Input: part model. Units: mm. Frame: model coordinates. A direction names the side the tool comes from. Give positions to 0.01 mm unless a question says otherwise; leave off trailing zeros. Write each loop counter-clockwise with the first axis right and the second up, starting at its lowest first coordinate (ties: lowest second). Pieces come first, ordered by that corner, then holes. Notation, with made-up numbers: (10.25, 41.25) -> (40.25, 41.25) arc R22 ccw to (40.25, 69.25) -> close; hole circle Ø7 at (-31, -18.75). An arc over 180 degrees is marked (long way). Answer as a JSON object with one key per item and string values. Group by question number.
from build123d import *

# Parameters (mm, degrees)
F1_DEPTH = 30
F4_DEPTH = 51.5
F5_DEPTH = 53.5
F6_DEPTH = 45
F7_DEPTH = 3


with BuildPart() as f1:
    # F0 (on Top) → F1 (new body)
    with BuildSketch(Plane.XY):
        with BuildLine():
            Line((92.1, -37.1), (90, -37.1))
            Line((90, -37.1), (70.1, -37.1))
            Line((70.1, -37.1), (55.207107, -37.1))
            Line((55.207107, -37.1), (58.096194, -39.989087))
            ThreePointArc((58.096194, -39.989087), (58.421353, -40.475722), (58.535534, -41.049747))
            Line((58.535534, -41.049747), (58.535534, -41.635534))
            ThreePointArc((58.535534, -41.635534), (58.096194, -42.696194), (57.035534, -43.135534))
            Line((57.035534, -43.135534), (43.964466, -43.135534))
            ThreePointArc((43.964466, -43.135534), (42.903806, -42.696194), (42.464466, -41.635534))
            Line((42.464466, -41.635534), (42.464466, -41.049747))
            ThreePointArc((42.464466, -41.049747), (42.578647, -40.475722), (42.903806, -39.989087))
            Line((42.903806, -39.989087), (45.792893, -37.1))
            Line((45.792893, -37.1), (45, -37.1))
            Line((45, -37.1), (26.284599, -37.1))
            Line((26.284599, -37.1), (29.173687, -39.989087))
            ThreePointArc((29.173687, -39.989087), (29.498846, -40.475722), (29.613026, -41.049747))
            Line((29.613026, -41.049747), (29.613026, -41.635534))
            ThreePointArc((29.613026, -41.635534), (29.173687, -42.696194), (28.113026, -43.135534))
            Line((28.113026, -43.135534), (15.041959, -43.135534))
            ThreePointArc((15.041959, -43.135534), (13.981298, -42.696194), (13.541959, -41.635534))
            Line((13.541959, -41.635534), (13.541959, -41.049747))
            ThreePointArc((13.541959, -41.049747), (13.656139, -40.475722), (13.981298, -39.989087))
            Line((13.981298, -39.989087), (16.870386, -37.1))
            Line((16.870386, -37.1), (12, -37.1))
            Line((12, -37.1), (12, -77.1))
            Line((12, -77.1), (125.1, -77.1))
            Line((125.1, -77.1), (125.1, -37.1))
            Line((125.1, -37.1), (92.1, -37.1))
        make_face()
    extrude(amount=F1_DEPTH)

    # F3 (on offset) → F4 (cut, symmetric)
    with BuildSketch(Plane.YZ.offset(68.5)):
        Polygon((-52.029371, 26.9), (-45.2, 0), (-45.2, 26.9), align=None)
        Polygon((-77.2, 0), (-45.2, 0), (-70.498638, 26.9), (-77.2, 26.9), align=None)
        Polygon((-70.498638, 26.9), (-45.2, 0), (-52.029371, 26.9), align=None)
    extrude(amount=F4_DEPTH, both=True, mode=Mode.SUBTRACT)

    # F3 (on offset) → F5 (join, symmetric)
    with BuildSketch(Plane.YZ.offset(68.5)):
        Polygon((-52.029371, 26.9), (-45.2, 0), (-45.2, 26.9), align=None)
        Polygon((-70.498638, 26.9), (-45.2, 0), (-52.029371, 26.9), align=None)
    extrude(amount=F5_DEPTH, both=True)

    # F3 (on offset) → F6 (cut, symmetric)
    with BuildSketch(Plane.YZ.offset(68.5)):
        Polygon((-70.498638, 26.9), (-45.2, 0), (-52.029371, 26.9), align=None)
    extrude(amount=F6_DEPTH, both=True, mode=Mode.SUBTRACT)

    # F3 (on offset) → F7 (join, symmetric)
    with BuildSketch(Plane.YZ.offset(68.5)):
        Polygon((-52.029371, 26.9), (-45.2, 0), (-45.2, 26.9), align=None)
        Polygon((-70.498638, 26.9), (-45.2, 0), (-52.029371, 26.9), align=None)
    extrude(amount=F7_DEPTH, both=True)


solid = f1.part
1. Section A-A (x = 100). Return the cut outline in (y, z).
2. Section D-D (y = -54). Return the cut outline in (x, z).
3. Section B-B (y = -65.5). Return the cut outline in (x, z), plus the area to 3 significant figures.
4. Reachability of faces 1 (the face through (69, -73, 26.9)), 2 (the face through (91, -37.1, 15)), 3 (the face through (22, -43.136, 15)) from +Z, -Z, +X, -X, +Y, -Y: full face, straight path, thin tool, end or side. Return the list, or none.
5. Contact query for flat-ended pins moving along their axis: pin 1 Ø6.5 at (x, z) = (48.5, 12.5) entering from +Y; pin 2 Ø12.5 at (x, y) = (69.5, -60) entering from -Z; pin 3 Ø8 at (x, z) = (50, 3) entering from -Y; pin 4 Ø4 at (x, z) = (66, 22.5) entering from -Y. Output: stop coordinate, or through.
6. Mould query, pull axis Y, two halves, no side actions, for faces 4 (the face through (116.8, -58.03, 13.64)), 5 (the face through (51, -43.136, 15)), 6 (the face through (36, -37.1, 15)), 7 (the face through (120, -65, 11)). Classes: pulls with the +Y half, pulls with the -Y half, needs draft (parallel to the pull), parting line crosses it, or undercut.
7. Line query: line 1 (X direction, y = -69, z = 20.5); line 2 (Z direction, x = 37.5, y = -74); line 3 (Y direction, x = 87, z = 22). Output: solid intervals per line, ascending.
8. Section C-C (x = 52). Return the cut outline in (y, z).
Working result:
{
 "1": {"outline": "(-77.1, 26.9) -> (-52.03, 26.9) -> (-45.2, 0) -> (-37.1, 0) -> (-37.1, 30) -> (-77.1, 30) -> close"},
 "2": {"outline": "(12, 0) -> (17, 0) -> (17, 9.36) -> (23.5, 9.36) -> (23.5, 26.9) -> (65.5, 26.9) -> (65.5, 9.36) -> (71.5, 9.36) -> (71.5, 26.9) -> (113.5, 26.9) -> (113.5, 9.36) -> (120, 9.36) -> (120, 0) -> (125.1, 0) -> (125.1, 30) -> (12, 30) -> close"},
 "3": {"outline": "(12, 0) -> (17, 0) -> (17, 21.58) -> (23.5, 21.58) -> (23.5, 26.9) -> (65.5, 26.9) -> (65.5, 21.58) -> (71.5, 21.58) -> (71.5, 26.9) -> (113.5, 26.9) -> (113.5, 21.58) -> (120, 21.58) -> (120, 0) -> (125.1, 0) -> (125.1, 30) -> (12, 30) -> close", "area": "723 mm^2"},
 "4": {"face 1": "-Z, -Y", "face 2": "+Z, -Z, +X, -X, +Y", "face 3": "+Z, -Z"},
 "5": {"pin 1": "stops at y = -37.1", "pin 2": "stops at z = 9.09", "pin 3": "stops at y = -46.98", "pin 4": "stops at y = -68.24"},
 "6": {"face 4": "pulls with the -Y half", "face 5": "undercut", "face 6": "pulls with the +Y half", "face 7": "needs draft"},
 "7": {"line 1": "x = 12 to 17, 120 to 125.1", "line 2": "z = 26.9 to 30", "line 3": "y = -50.79 to -37.1"},
 "8": {"outline": "(-77.1, 26.9) -> (-52.03, 26.9) -> (-45.2, 0) -> (-43.14, 0) -> (-43.14, 30) -> (-77.1, 30) -> close"}
}
